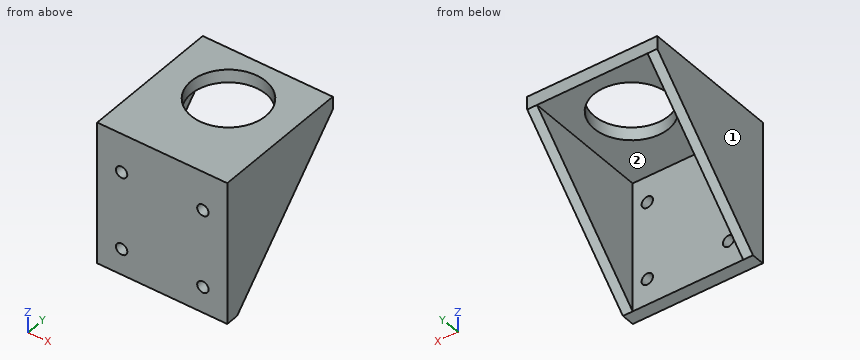
```python
from build123d import *

# Parameters (mm, degrees)
SKETCH_1_W           = 34
SKETCH_1_H           = 51
EXTRUDE_1_DEPTH      = 4
SKETCH_2_R           = 11.5
CUT_EXTRUDE_1_DEPTH  = 31.907118921
SKETCH_5_W           = 34
SKETCH_5_H           = 15
EXTRUDE_2_DEPTH      = 4
SKETCH_6_R           = 1.5
CUT_EXTRUDE_3_DEPTH  = 4
SKETCH_12_W          = 34
SKETCH_12_H          = 4
CUT_EXTRUDE_5_DEPTH  = 5
SKETCH_13_W          = 34
SKETCH_13_H          = 4
CUT_EXTRUDE_6_DEPTH  = 7
SKETCH_14_W          = 34
SKETCH_14_H          = 4
EXTRUDE_3_DEPTH      = 33
SKETCH_15_R          = 1.75
CUT_EXTRUDE_7_DEPTH  = 44
EXTRUDE_4_DEPTH      = 3
EXTRUDE_5_DEPTH      = 3
SKETCH_18_R          = 1.75
EXTRUDE_6_DEPTH      = 4
EXTRUDE_7_DEPTH      = 5
SKETCH_20_W          = 63.510352062
SKETCH_20_H          = 72.285945639
CUT_EXTRUDE_10_DEPTH = 67
SKETCH_21_W          = 4
SKETCH_21_H          = 43
EXTRUDE_8_DEPTH      = 3
SKETCH_22_W          = 4
SKETCH_22_H          = 43
EXTRUDE_9_DEPTH      = 3
SKETCH_23_W          = 40
SKETCH_23_H          = 4
EXTRUDE_10_DEPTH     = 40
SKETCH_24_W          = 3
SKETCH_24_H          = 39
EXTRUDE_11_DEPTH     = 40
CUT_EXTRUDE_11_DEPTH = 72.5
SKETCH_26_R          = 1.75
CUT_EXTRUDE_12_DEPTH = 5


with BuildPart() as part:
    # 草图1 → 凸台-拉伸1 (new body)
    with BuildSketch(Plane.XY):
        Rectangle(SKETCH_1_W, SKETCH_1_H)
    extrude(amount=EXTRUDE_1_DEPTH)

    # 草图2 → 切除-拉伸1 (cut, through all)
    with BuildSketch(Plane.XY.offset(4)):
        with Locations((0, -2.5)):
            Circle(SKETCH_2_R)
    extrude(amount=-CUT_EXTRUDE_1_DEPTH, mode=Mode.SUBTRACT)

    # 草图5 → 凸台-拉伸2 (add)
    with BuildSketch(Plane.XZ.offset(25.5)):
        with Locations((0, 7.5)):
            Rectangle(SKETCH_5_W, SKETCH_5_H)
    extrude(amount=EXTRUDE_2_DEPTH)

    # 草图6 → 切除-拉伸3 (cut)
    with BuildSketch(Plane.XZ.offset(29.5)):
        with Locations(Location((13, 7.5, 0), (0, 0, 270))):
            Circle(SKETCH_6_R)
        with Locations(Location((-13, 7.5, 0), (0, 0, 90))):
            Circle(SKETCH_6_R)
    extrude(amount=-CUT_EXTRUDE_3_DEPTH, mode=Mode.SUBTRACT)

    # 草图12 → 切除-拉伸5 (cut)
    with BuildSketch(Plane(origin=(0, 25.5, 0), x_dir=(1, 0, 0), z_dir=(0, 1, 0))):
        with Locations((0, -2)):
            Rectangle(SKETCH_12_W, SKETCH_12_H)
    extrude(amount=-CUT_EXTRUDE_5_DEPTH, mode=Mode.SUBTRACT)

    # 草图13 → 切除-拉伸6 (cut)
    with BuildSketch(Plane(origin=(0, 20.5, 0), x_dir=(1, 0, 0), z_dir=(0, 1, 0))):
        with Locations((0, -2)):
            Rectangle(SKETCH_13_W, SKETCH_13_H)
    extrude(amount=-CUT_EXTRUDE_6_DEPTH, mode=Mode.SUBTRACT)

    # 草图14 → 凸台-拉伸3 (add)
    with BuildSketch(Plane.XY.offset(15)):
        with Locations((0, -27.5)):
            Rectangle(SKETCH_14_W, SKETCH_14_H)
    extrude(amount=EXTRUDE_3_DEPTH)

    # 草图15 → 切除-拉伸7 (cut)
    with BuildSketch(Plane(origin=(0, -25.5, 0), x_dir=(1, 0, 0), z_dir=(0, 1, 0))):
        with Locations(Location((13, -40.5, 0), (0, 0, 270))):
            Circle(SKETCH_15_R)
        with Locations(Location((-13, -40.5, 0), (0, 0, 270))):
            Circle(SKETCH_15_R)
    extrude(amount=-CUT_EXTRUDE_7_DEPTH, mode=Mode.SUBTRACT)

    # 草图16 → 凸台-拉伸4 (add)
    with BuildSketch(Plane.ZY.offset(17)):
        Polygon((4, -25.5), (4, -6), (24, -25.5), align=None)
    extrude(amount=-EXTRUDE_4_DEPTH)

    # 草图17 → 凸台-拉伸5 (add)
    with BuildSketch(Plane(origin=(17, 0, 0), x_dir=(0, 0, -1), z_dir=(1, 0, 0))):
        Polygon((-24, -25.5), (-4, -6), (-4, -25.5), align=None)
    extrude(amount=-EXTRUDE_5_DEPTH)

    # 草图18 → 凸台-拉伸6 (add)
    with BuildSketch(Plane(origin=(0, -25.5, 0), x_dir=(1, 0, 0), z_dir=(0, 1, 0))):
        with BuildLine():
            Line((20.499000769, -32.499999751), (17, -24))
            Line((17, -24), (-17, -24))
            Line((-17, -24), (-20.500999231, -32.499999751))
            Line((-20.500999231, -32.499999751), (-20.500999231, -40.499999751))
            ThreePointArc((-20.500999231, -40.499999751), (-17.718513652, -47.217514172), (-11.000999231, -49.999999751))
            Line((-11.000999231, -49.999999751), (10.999000769, -49.999999751))
            ThreePointArc((10.999000769, -49.999999751), (17.71651519, -47.217514172), (20.499000769, -40.499999751))
            Line((20.499000769, -40.499999751), (20.499000769, -32.499999751))
        make_face()
        with Locations(Location((-13, -40.5, 0), (0, 0, 270))):
            Circle(SKETCH_18_R, mode=Mode.SUBTRACT)
        with Locations(Location((13, -40.5, 0), (0, 0, 270))):
            Circle(SKETCH_18_R, mode=Mode.SUBTRACT)
    extrude(amount=-EXTRUDE_6_DEPTH)

    # 草图19 → 凸台-拉伸7 (add)
    with BuildSketch(Plane(origin=(0, -25.5, 0), x_dir=(1, 0, 0), z_dir=(0, 1, 0))):
        Polygon((-20.500999231, -32.499999751), (-17.500999231, -32.499999751), (-14, -24), (-14, -16), (-17, -16), (-17, -24), align=None)
        Polygon((17, -24), (20.499000769, -32.499999751), (17.499000769, -32.499999751), (14, -24), (14, -16), (17, -16), align=None)
    extrude(amount=EXTRUDE_7_DEPTH)

    # 草图20 → 切除-拉伸10 (cut)
    with BuildSketch(Plane.XY.offset(4)):
        with Locations((0, -7.757033155)):
            Rectangle(SKETCH_20_W, SKETCH_20_H)
    extrude(amount=CUT_EXTRUDE_10_DEPTH, mode=Mode.SUBTRACT)

    # 草图21 → 凸台-拉伸8 (add)
    with BuildSketch(Plane(origin=(17, 0, 0), x_dir=(0, 0, -1), z_dir=(1, 0, 0))):
        with Locations((-2, -8)):
            Rectangle(SKETCH_21_W, SKETCH_21_H)
    extrude(amount=EXTRUDE_8_DEPTH)

    # 草图22 → 凸台-拉伸9 (add)
    with BuildSketch(Plane.ZY.offset(17)):
        with Locations((2, -8)):
            Rectangle(SKETCH_22_W, SKETCH_22_H)
    extrude(amount=EXTRUDE_9_DEPTH)

    # 草图23 → 凸台-拉伸10 (add)
    with BuildSketch(Plane(origin=(0, 0, 0), x_dir=(-1, 0, 0), z_dir=(0, 0, -1))):
        with Locations((0, -27.5)):
            Rectangle(SKETCH_23_W, SKETCH_23_H)
    extrude(amount=EXTRUDE_10_DEPTH)

    # 草图24 → 凸台-拉伸11 (add)
    with BuildSketch(Plane(origin=(0, 0, 0), x_dir=(-1, 0, 0), z_dir=(0, 0, -1))):
        with Locations((18.5, -6)):
            Rectangle(SKETCH_24_W, SKETCH_24_H)
        with Locations((-18.5, -6)):
            Rectangle(SKETCH_24_W, SKETCH_24_H)
    extrude(amount=EXTRUDE_11_DEPTH)

    # 草图25 → 切除-拉伸11 (cut, symmetric)
    with BuildSketch(Plane(origin=(-17, 0, 0), x_dir=(0, 0, -1), z_dir=(1, 0, 0))):
        Polygon((0, 13.5), (40, -25.5), (40, 13.5), align=None)
    extrude(amount=CUT_EXTRUDE_11_DEPTH, both=True, mode=Mode.SUBTRACT)

    # 草图26 → 切除-拉伸12 (cut)
    with BuildSketch(Plane(origin=(0, -25.5, 0), x_dir=(1, 0, 0), z_dir=(0, 1, 0))):
        with Locations(Location((-12.5, 32, 0), (0, 0, 270))):
            Circle(SKETCH_26_R)
        with Locations(Location((12.5, 32, 0), (0, 0, 270))):
            Circle(SKETCH_26_R)
        with Locations(Location((12.5, 8, 0), (0, 0, 270))):
            Circle(SKETCH_26_R)
        with Locations(Location((-12.5, 8, 0), (0, 0, 270))):
            Circle(SKETCH_26_R)
    extrude(amount=-CUT_EXTRUDE_12_DEPTH, mode=Mode.SUBTRACT)


solid = part.part
```
Work out the finished part from the listing and answer in its coordinate system (mm). Face numbers are marked on the shaded views. A direction names the side the tool comes from. Coordinates: 2 decimals unless noted, no trailing zeros. Loops run counter-clockwise (first coordinate to the right, second up) from the corner with the lowest first, then second, coordinate; pieces in that order, holes last. Notation, with made-up numbers: (-22.75, -2.5) -> (30.25, -2.5) arc R6 ccw to (30.25, 6.5) -> close; hole circle Ø6 at (24, -31.5). An arc over 180 degrees is marked (long way). Answer as CSV lines item,"result".
Q1. The part is cut by section D-D on y = -13. Write down the section's boundary in (x, z).
Findings:
outline,"(-20, -27.18) -> (-17, -27.18) -> (-17, 0) -> (-4.69, 0) -> (-4.69, 4) -> (-20, 4) -> close; (4.69, 0) -> (17, 0) -> (17, -27.18) -> (20, -27.18) -> (20, 4) -> (4.69, 4) -> close"
Q2. The part is cut by section B-B on z = -8. Write down the section's boundary in (x, y).
Findings:
outline,"(-20, -29.5) -> (-14.25, -29.5) -> (-14.25, -25.5) -> (-17, -25.5) -> (-17, 5.7) -> (-20, 5.7) -> close; (-10.75, -29.5) -> (10.75, -29.5) -> (10.75, -25.5) -> (-10.75, -25.5) -> close; (14.25, -29.5) -> (20, -29.5) -> (20, 5.7) -> (17, 5.7) -> (17, -25.5) -> (14.25, -25.5) -> close"
Q3. Find the intervals of material crossed by probe 1 along X at (y, z) = (-26.7, -32); probe 2 along X at (y, z) = (-12, -20.5); probe 3 along Y at (x, z) = (0, 3.25), in increasing order.
Findings:
probe 1,"x = -20 to -14.25, -10.75 to 10.75, 14.25 to 20"
probe 2,"x = -20 to -17, 17 to 20"
probe 3,"y = -29.5 to -14, 9 to 13.5"
Q4. This flat-tipped pin is pushed along its axis until it touches: pin 1 (17 mm diameter, centred on x = 1.5, z = -25.5, fed in from +Y). Where does it stop, or does it pass through?
Findings:
pin 1,"stops at y = -25.5"
Q5. A tool of negligible diameter and unlimited length cuts with its end or side. For the marked faces 1 and 2, from which of +Z, -Z, +X, -X, +Y, -Y can it reach the whole face along a straight path? Write none if from no direction.
Findings:
face 1,"+Z, -Z, -X, +Y, -Y"
face 2,"-Z, +Y"
Q6. The part is cut by section C-C on x = 12.5. Write down the section's boundary in (y, z).
Findings:
outline,"(-29.5, -40) -> (-25.5, -40) -> (-25.5, -33.75) -> (-29.5, -33.75) -> close; (-29.5, -30.25) -> (-25.5, -30.25) -> (-25.5, -9.75) -> (-29.5, -9.75) -> close; (-29.5, -6.25) -> (-25.5, -6.25) -> (-25.5, 0) -> (13.5, 0) -> (13.5, 4) -> (-29.5, 4) -> close"
Q7. The part is cut by section A-A on x = 0. Write down the section's boundary in (y, z), and give its area (3 significant figures).
Findings:
outline,"(-29.5, -40) -> (-25.5, -40) -> (-25.5, 0) -> (-14, 0) -> (-14, 4) -> (-29.5, 4) -> close; (9, 0) -> (13.5, 0) -> (13.5, 4) -> (9, 4) -> close"
area,"240 mm²"
